Here's the drawing with two shaded views (mm, measured from the low corner). I have some questions. Round coordinates to 2 decimals unless told otherwise and drop trailing zeros. Order: outer loops, then holes, each group sorted by start corner. A loop starts at its lowest first (then second) coordinate and runs counter-clockwise, first axis right, second up.
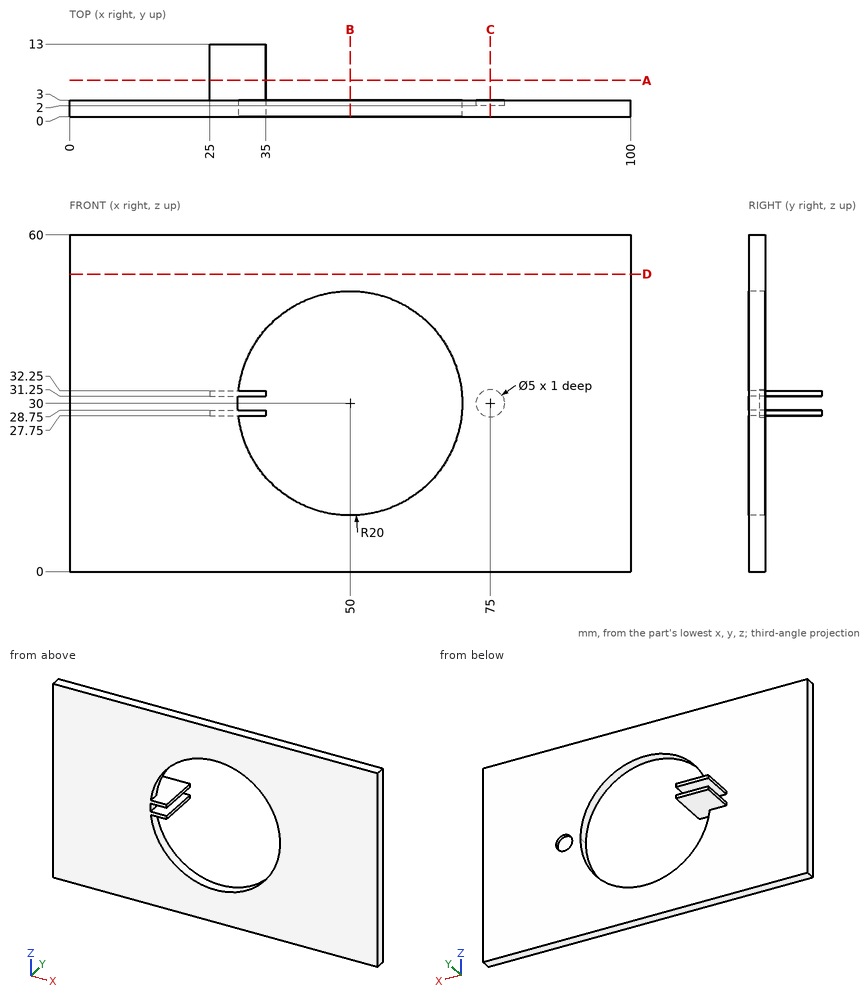
1. I'm going to push flat-ended pins straight in: P1, Ø0.8, axis at y = 7.5, z = 28.5, coming from the -X side; P2, Ø8, axis at x = 15.5, z = 42, coming from the +Y side; P3, Ø8, axis at x = 16, z = 21.5, coming from the -Y side; P4, Ø0.8, axis at y = 4.5, z = 28.5, coming from the +X side. Where does each tip first touch, or does it pass through?
Evaluation:
P1: stops at x = 25
P2: stops at y = 3
P3: stops at y = 0
P4: stops at x = 35
2. If we section it at C-C, the plane x = 75: Write out the boundary of the cut face in (y, z).
Evaluation:
outline: (0, 0) - (3, 0) - (3, 27.5) - (2, 27.5) - (2, 32.5) - (3, 32.5) - (3, 60) - (0, 60) - close
3. I need wall thicknesses on probe 1 along X at (y, z) = (2.35, 30); probe 2 along Z at (x, y) = (75, 2.4); probe 3 along Y at (x, z) = (41.5, 50). Which ranges of each line are inside material? Lowest first, please.
Evaluation:
probe 1: x = 0 to 30, 70 to 72.5, 77.5 to 100
probe 2: z = 0 to 27.5, 32.5 to 60
probe 3: y = 0 to 3
4. If we section it at D-D, the plane z = 53: Write out the boundary of the cut face in (x, y).
Evaluation:
outline: (0, 0) - (100, 0) - (100, 3) - (0, 3) - close
5. If we section it at B-B, the plane x = 50: Write out the boundary of the cut face in (y, z).
Evaluation:
outline: (0, 0) - (3, 0) - (3, 10) - (0, 10) - close; (0, 50) - (3, 50) - (3, 60) - (0, 60) - close
6. If we section it at A-A, the plane y = 6.5: Write out the boundary of the cut face in (x, z), and give its area (3 significant figures).
Evaluation:
outline: (25, 27.75) - (35, 27.75) - (35, 28.75) - (25, 28.75) - close; (25, 31.25) - (35, 31.25) - (35, 32.25) - (25, 32.25) - close
area: 20.0 mm2
